The model under review builds one solid part; all positions refer to its coordinate system, in mm. Round coordinates to 2 decimals unless told otherwise and drop trailing zeros. Loops run counter-clockwise (first coordinate to the right, second up) from the corner with the lowest first, then second, coordinate; pieces in that order, holes last. Notation, with made-up numbers: (79, 4) - (138, 4) arc R24 cw to (138, 21) - close; hole circle Ø9 at (-19, 79). An arc over 180 degrees is marked (long way). Answer as CSV lines item,"result".
from build123d import *

# Parameters (mm, degrees)
F0_R          = 0.75
F1_DEPTH      = 40
F1_DEPTH_BACK = 5
F4_DEPTH      = 28.8156013334
F4_DEPTH_BACK = 4.0668639918
F6_W          = 6.4407079129
F6_H          = 2.7354915243
F7_DEPTH      = 0.869841948
F7_DEPTH_BACK = 39.5235462537


with BuildPart() as f1:
    # F0 (on Top) → F1 (new body, two sides)
    with BuildSketch(Plane.XY) as f1_sk:
        Circle(F0_R)
    extrude(amount=F1_DEPTH)
    extrude(f1_sk.sketch, amount=-F1_DEPTH_BACK)

    # F3 (on line) → F4 (cut, two sides)
    with BuildSketch(Plane(origin=(0, 0, 0), x_dir=(1, 0, 0), z_dir=(0, 0.7071067812, -0.7071067812))) as f4_sk:
        Polygon((-3.5966049702, -6.2295025431), (0, 0), (3.5966049702, -6.2295025431), (3.5966049702, 7.7731425289), (-3.5966049702, 7.7731425289), align=None)
    extrude(amount=-F4_DEPTH, mode=Mode.SUBTRACT)
    extrude(f4_sk.sketch, amount=F4_DEPTH_BACK, mode=Mode.SUBTRACT)

    # F6 (on face) → F7 (cut, two sides)
    with BuildSketch(Plane(origin=(0, 0, 0), x_dir=(1, 0, 0), z_dir=(0, -0.1736481777, -0.984807753))) as f7_sk:
        with Locations((-0.1402113121, -2.0677457621)):
            Rectangle(F6_W, F6_H)
    extrude(amount=F7_DEPTH, mode=Mode.SUBTRACT)
    extrude(f7_sk.sketch, amount=-F7_DEPTH_BACK, mode=Mode.SUBTRACT)


solid = f1.part
1. Take a section at B-B (y = 0.3). State the section outline as (x, z) points.
Numbers:
outline,"(-0.69, 1.38) - (0, -0.3) - (0.69, 1.38) - (0.69, 40) - (-0.69, 40) - close"
2. Take a section at A-A (z = 26.5). State the section outline as (x, y) points.
Numbers:
outline,"circle Ø1.5 at (0, 0)"
3. Wall thickness on probe 1 along X at (y, z) = (-0.1, 25.5); probe 2 along Y at (x, z) = (0.45, 18); probe 3 along Z at (x, y) = (0.15, 0.15): over which ranges is each line inside the solid? List them lowest first.
Numbers:
probe 1,"x = -0.74 to 0.74"
probe 2,"y = -0.6 to 0.6"
probe 3,"z = 0.22 to 40"
